from build123d import *

# Parameters (mm, degrees)
BOSS_EXTRUDE1_DEPTH = 12
FILLET1_R           = 1
FILLET2_R           = 1
FILLET3_R           = 0.25


with BuildPart() as part:
    # Sketch1 → Boss-Extrude1 (new body)
    with BuildSketch(Plane.XY):
        with BuildLine():
            Line((6.738137725, -6.88), (4.878137725, -6.88))
            Line((4.878137725, -6.88), (4.531835438, -5.38))
            ThreePointArc((4.531835438, -5.38), (7.034339517, 0), (4.531835438, 5.38))
            Line((4.531835438, 5.38), (4.878137725, 6.88))
            Line((4.878137725, 6.88), (6.738137725, 6.88))
            ThreePointArc((6.738137725, 6.88), (9.63, 0), (6.738137725, -6.88))
        make_face()
    extrude(amount=BOSS_EXTRUDE1_DEPTH)

    # Fillet1
    fillet1_edges = [part.edges().sort_by_distance(p)[0] for p in [
        (4.531835438, -5.38, 6),
        (4.531835438, 5.38, 6),
    ]]
    fillet(fillet1_edges, radius=FILLET1_R)

    # Fillet2
    fillet2_edges = [part.edges().sort_by_distance(p)[0] for p in [
        (5.808137725, -6.88, 0),
        (5.808137725, 6.88, 0),
        (5.808137725, -6.88, 12),
        (5.808137725, 6.88, 12),
    ]]
    fillet(fillet2_edges, radius=FILLET2_R)

    # Fillet3
    fillet3_edges = [part.edges().sort_by_distance(p)[0] for p in [
        (7.034339517, 0, 0),
        (4.687877266, 5.411310183, 0),
        (7.034339517, 0, 12),
        (4.687877266, -5.411310183, 12),
        (6.738137725, -6.88, 6),
        (4.878137725, -6.88, 6),
        (9.63, 0, 0),
        (6.738137725, 6.88, 6),
        (9.63, 0, 12),
        (7.064336577, 6.544619807, 11.7471817),
        (7.064336589, -6.544619821, 11.747181705),
        (7.064336577, 6.544619807, 0.2528183),
        (7.064336577, -6.544619807, 0.2528183),
        (4.687877266, -5.411310183, 0),
        (4.655934772, -5.914769545, 11.999395357),
        (4.655934772, -5.914769545, 0.000604643),
        (4.815123489, -6.607055355, 11.686578845),
        (4.815123489, -6.607055355, 0.313421155),
        (4.878137725, 6.88, 6),
        (4.815123489, 6.607055355, 11.686578845),
        (4.815123489, 6.607055355, 0.313421155),
        (4.687877266, 5.411310183, 12),
        (4.655934776, 5.914769544, 11.99939535),
        (4.655934776, 5.914769544, 0.00060465),
    ]]
    fillet(fillet3_edges, radius=FILLET3_R)


solid = part.part
Could you check a few things on this model? Use its own coordinates, in mm. Give positions to 0.01 mm unless a question says otherwise; leave off trailing zeros. Write each loop counter-clockwise with the first axis right and the second up, starting at its lowest first coordinate (ties: lowest second). Pieces come first, ordered by that corner, then holes. Notation, with made-up numbers: (9, -11) -> (21, -11) arc R25 ccw to (21, 9) -> close; hole circle Ø4 at (-23, 57). An arc over 180 degrees is marked (long way). Answer as CSV lines item,"result". Start each with the question number.
(1) If we mould it in two halves opening along Y, with no side actions, what happens to faces 1 (the face through (8, 0, 0)), 2 (the face through (9.63, 0.11, 5.92)), 3 (the face through (6.089, -6.595, 11.699)), 4 (the face through (4.675, -5.452, 6.08))? For each: +Y half, -Y half, draft (parallel to the pull), parting line (faces both ways), or undercut.
(2) Please list where these lines run through material, in increasing order: line 1 (Y direction, x = 5.75, z = 0.5); line 2 (X direction, y = 0, z = 9.75); line 3 (Y direction, x = 6, z = 9.5).
(3) If we section it at A-A, the plane z = 9.75: Write out the boundary of the cut face in (x, y), and give its area (3 significant figures).
(4) I'm going to push flat-ended pins straight in: pin 1 Ø1 at (y, z) = (2.5, 9) entering from +X; pin 2 Ø3 at (y, z) = (-2.5, 7.5) entering from +X; pin 3 Ø4 at (y, z) = (-1, 1.5) entering from -X. Where does each tip first touch, or does it pass through?
Answer list:
1,face 1,"draft"
1,face 2,"parting line"
1,face 3,"-Y half"
1,face 4,"undercut"
2,line 1,"-6.75 to -4.05, 4.05 to 6.75"
2,line 2,"7.03 to 9.63"
2,line 3,"-6.88 to -3.67, 3.67 to 6.88"
3,outline,"(4.66, -5.95) -> (4.83, -6.69) arc R0.25 ccw to (5.08, -6.88) -> (6.64, -6.88) arc R0.25 ccw to (6.81, -6.81) arc R9.63 ccw to (6.81, 6.81) arc R0.25 ccw to (6.64, 6.88) -> (5.08, 6.88) arc R0.25 ccw to (4.83, 6.69) -> (4.66, 5.95) arc R1 ccw to (4.94, 5.01) arc R7.03 cw to (4.94, -5.01) arc R1 ccw to start"
3,area,"38.5 mm^2"
4,pin 1,"x = 9.42"
4,pin 2,"x = 9.58"
4,pin 3,"x = 6.36"
